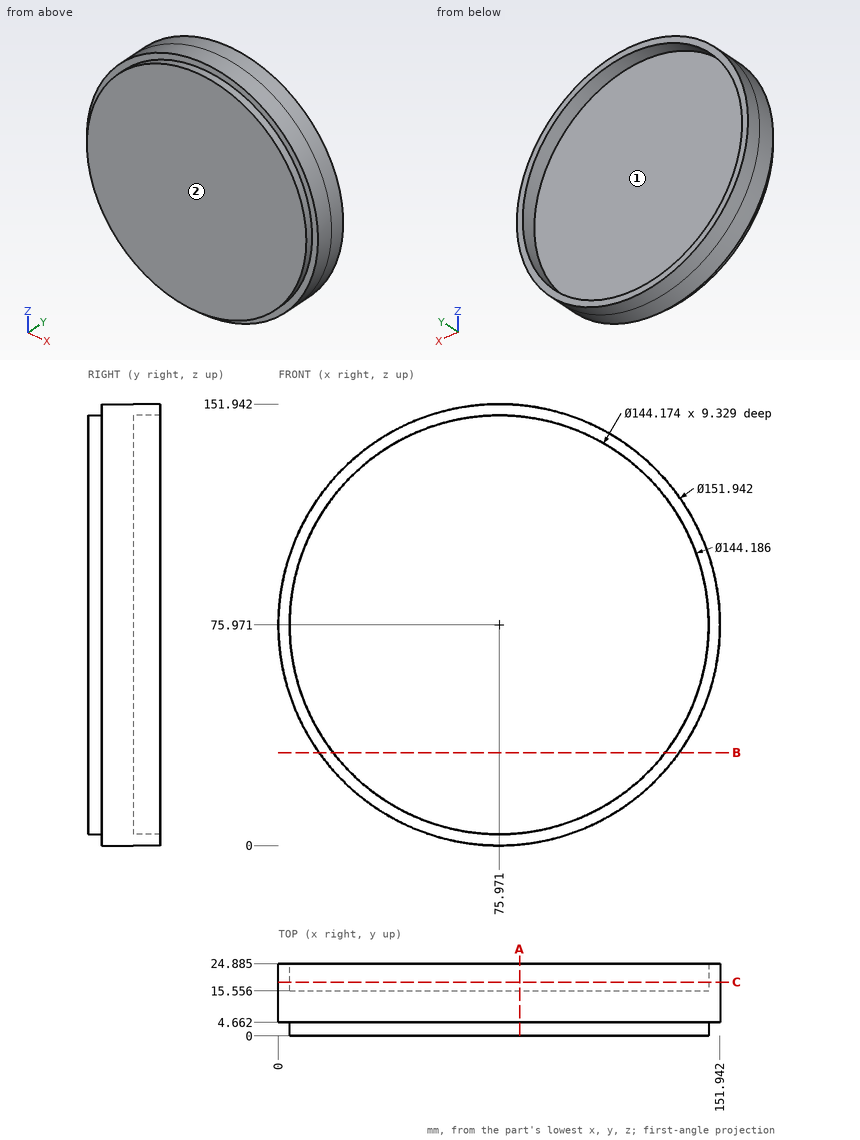
For this review, use the dimensioned drawing (mm, ordinates from the lowest corner) and the shaded views. Give positions to 0.01 mm unless a question says otherwise; leave off trailing zeros. Order: outer loops, then holes, each group sorted by start corner. A loop starts at its lowest first (then second) coordinate and runs counter-clockwise, first axis right, second up. Notation, with made-up numbers: (65, 11) - (75, 11) arc R18 ccw to (75, 27) - close; hole circle Ø7 at (-24.75, 64). An arc over 180 degrees is marked (long way). Use CSV: the item, a comma, the result in double quotes. Start each with the question number.
Q1. Draft analysis for pull direction Z (two halves, no side actions). For the marked faces 1 and 2, state which applies: pulls with the +Z half, pulls with the -Z half, needs draft (parallel to the pull), parting line crosses it, or undercut.
Q2. Take a section at B-B (z = 32). State the section outline as (x, y) points (1 decimal), and give its area (3 significant figures).
Q3. For P1, Ø8, axis at x = 123.5, z = 40, coming from the -Y side; P2, Ø12, axis at y = 17.5, z = 51, coming from the -X side; P3, Ø12, axis at x = 66.5, y = 12.5, coming from the -Z side; P4, Ø6, axis at x = 102.5, z = 101.5, coming from the +Y side, all flat-tipped, find the tip position at first contact; note any pin that passes through.
Q4. Take a section at C-C (y = 18.5). State the section outline as (x, z) points (1 decimal), and give its area (3 significant figures).
Q5. Take a section at A-A (x = 83). State the section outline as (y, z) points (1 decimal).
Q6. For line 1 (Z direction, x = 74, y = 23.5) (1 decimal); line 2 (Y direction, x = 36, z = 82.5); line 3 (X direction, y = 19.25, z = 118) (1 decimal), list the stretches that pass through material, from the lowest coordinate up.
Calculated:
1,face 1,"undercut"
1,face 2,"needs draft"
2,outline,"(14, 4.7) - (18.8, 4.7) - (18.8, 0) - (133.1, 0) - (133.1, 4.7) - (137.9, 4.7) - (137.9, 24.9) - (133.1, 24.9) - (133.1, 15.6) - (18.8, 15.6) - (18.8, 24.9) - (14, 24.9) - close"
2,area,"1,970 mm²"
3,P1,"stops at y = 0"
3,P2,"stops at x = 2.41"
3,P3,"stops at z = 0.08"
3,P4,"stops at y = 15.56"
4,outline,"circle Ø151.9 at (76, 76); hole circle Ø144.2 at (76, 76)"
4,area,"1,810 mm²"
5,outline,"(0, 4.2) - (4.7, 4.2) - (4.7, 0.3) - (24.9, 0.3) - (24.9, 4.2) - (15.6, 4.2) - (15.6, 147.7) - (24.9, 147.7) - (24.9, 151.6) - (4.7, 151.6) - (4.7, 147.7) - (0, 147.7) - close"
6,line 1,"z = 0 to 3.9, 148 to 151.9"
6,line 2,"y = 0 to 15.56"
6,line 3,"x = 12.7 to 17.4, 134.5 to 139.3"
